from build123d import *

# Parameters (mm, degrees)
F0_W     = 76.039264
F0_H     = 81
F0_W_2   = 72
F0_H_2   = 77
F0_R     = 1.9
F0_W_3   = 51
F0_H_3   = 71
F1_DEPTH = 1
F2_DEPTH = 25
F3_DEPTH = 8


with BuildPart() as f1:
    # F0 (on Top) → F1 (new body)
    with BuildSketch(Plane.XY):
        with Locations((0.69853, 0)):
            Rectangle(F0_W, F0_H)
        with Locations((0.69853, 0)):
            Rectangle(F0_W_2, F0_H_2, mode=Mode.SUBTRACT)
        with Locations((0.69853, 0)):
            Rectangle(F0_W_2, F0_H_2)
        with Locations((-27.50147, -32)):
            Circle(F0_R, mode=Mode.SUBTRACT)
        with Locations((31.89853, -32)):
            Circle(F0_R, mode=Mode.SUBTRACT)
        with Locations((-27.50147, 31)):
            Circle(F0_R, mode=Mode.SUBTRACT)
        with Locations((0.69853, 0)):
            Rectangle(F0_W_3, F0_H_3, mode=Mode.SUBTRACT)
        with Locations((31.89853, 31)):
            Circle(F0_R, mode=Mode.SUBTRACT)
        with Locations((31.89853, 31)):
            Circle(F0_R)
        with Locations((-27.50147, 31)):
            Circle(F0_R)
        with Locations((-27.50147, -32)):
            Circle(F0_R)
        with Locations((31.89853, -32)):
            Circle(F0_R)
    extrude(amount=F1_DEPTH)

    # F0 (on Top) → F2 (join)
    with BuildSketch(Plane.XY):
        with Locations((0.69853, 0)):
            Rectangle(F0_W, F0_H)
        with Locations((0.69853, 0)):
            Rectangle(F0_W_2, F0_H_2, mode=Mode.SUBTRACT)
    extrude(amount=F2_DEPTH)

    # F0 (on Top) → F3 (join)
    with BuildSketch(Plane.XY):
        with Locations((-27.50147, 31)):
            Circle(F0_R)
        with Locations((31.89853, 31)):
            Circle(F0_R)
        with Locations((-27.50147, -32)):
            Circle(F0_R)
        with Locations((31.89853, -32)):
            Circle(F0_R)
    extrude(amount=F3_DEPTH)


solid = f1.part
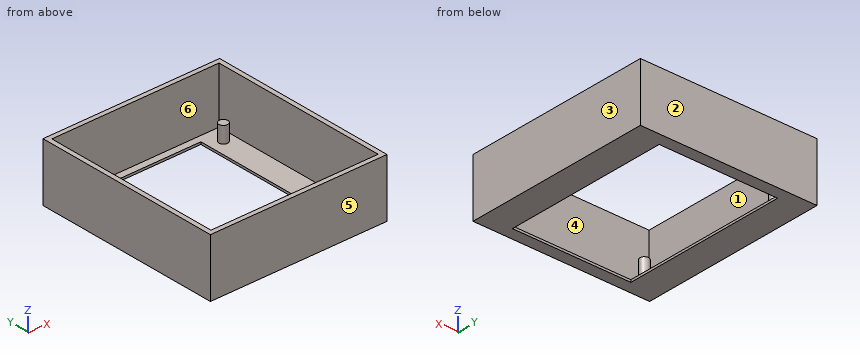
Design review of the part built by this model. Coordinates are the model's own, in mm. Face numbers are marked on the shaded views. A direction names the side the tool comes from. Coordinates: 2 decimals unless noted, no trailing zeros. Order: outer loops, then holes, each group sorted by start corner. A loop starts at its lowest first (then second) coordinate and runs counter-clockwise, first axis right, second up. Notation, with made-up numbers: (-34.5, 18.25) - (3.5, 18.25) arc R27 cw to (3.5, 55.25) - close; hole circle Ø10 at (64.5, 48.25). An arc over 180 degrees is marked (long way). Put each result on its own line as item: value.
1) Wall thickness on L1, parallel to Y at x = -9, z = 2.5; L2, parallel to X at y = 22, z = 21.25; L3, parallel to Y at x = -29, z = 2: over which ranges is each line inside the solid? List them lowest first. Write a range as from..to.
Response values:
L1: y = -40.5..-38.5, 38.5..40.5
L2: x = -37.32..-35.3, 36.7..38.72
L3: y = -40.5..-38.5, -33.17..-30.83, 29.83..32.17, 38.5..40.5
2) Insertion check: P1, Ø1.9, axis at x = -27, y = -32.5, coming from the +Z side; P2, Ø1.5, axis at x = 23.5, y = -17, coming from the -Z side. Each pin has a flat end and moves straight along its axis. Give the tip position at first contact, or say it passes through.
Response values:
P1: stops at z = 8
P2: passes through
3) Take a section at A-A, the plane z = 23.5. Give the boundary of the cut face in (x, y).
Response values:
outline: (-37.32, -40.5) - (38.72, -40.5) - (38.72, 40.5) - (-37.32, 40.5) - close; hole (-35.3, -38.5) - (36.7, -38.5) - (36.7, 38.5) - (-35.3, 38.5) - close
4) Take a section at B-B, the plane x = -1. Give the boundary of the cut face in (y, z), and give its area (3 significant figures).
Response values:
outline: (-40.5, 0) - (-35.5, 0) - (-35.5, 1) - (-38.5, 1) - (-38.5, 25) - (-40.5, 25) - close; (35.5, 0) - (40.5, 0) - (40.5, 25) - (38.5, 25) - (38.5, 1) - (35.5, 1) - close
area: 106 mm²
5) The part is to be moulded in two halves that separate along X. For the marked faces 3, 4, 5 and 6, say which applies: released by +X, released by -X, zero draft, split by the parting line, or undercut.
Response values:
face 3: released by +X
face 4: undercut
face 5: zero draft
face 6: undercut
6) Tool access review of the marked faces 1 and 2: name each direction out of +Z, -Z, +X, -X, +Y, -Y from which nothing blocks a thin tool from reaching the whole face with its end or side.
Response values:
face 1: +Z
face 2: +Z, -Z, +X, -X, +Y
7) Take a section at C-C, the plane y = 31. Give the boundary of the cut face in (x, z).
Response values:
outline: (-37.32, 0) - (-24.8, 0) - (-24.8, 1) - (-25.6, 1) - (-25.6, 8) - (-29.4, 8) - (-29.4, 1) - (-35.3, 1) - (-35.3, 25) - (-37.32, 25) - close; (26.2, 0) - (38.72, 0) - (38.72, 25) - (36.7, 25) - (36.7, 1) - (33.8, 1) - (33.8, 8) - (30, 8) - (30, 1) - (26.2, 1) - close
8) Take a section at D-D, the plane y = -12.5. Give the boundary of the cut face in (x, z), and give its area (3 significant figures).
Response values:
outline: (-37.32, 0) - (-24.8, 0) - (-24.8, 1) - (-35.3, 1) - (-35.3, 25) - (-37.32, 25) - close; (26.2, 0) - (38.72, 0) - (38.72, 25) - (36.7, 25) - (36.7, 1) - (26.2, 1) - close
area: 122 mm²
